The drawing under review shows one solid part. Ordinate dimensions are in mm from its lowest x, y, z. Give positions to 0.01 mm unless a question says otherwise; leave off trailing zeros. Loops run counter-clockwise (first coordinate to the right, second up) from the corner with the lowest first, then second, coordinate; pieces in that order, holes last. Notation, with made-up numbers: (-34, -23.75) - (25, -23.75) arc R15 cw to (25, -12.75) - close; hole circle Ø3 at (44, 77). An arc over 180 degrees is marked (long way). Write each question's results on one line, items separated by ' | '.
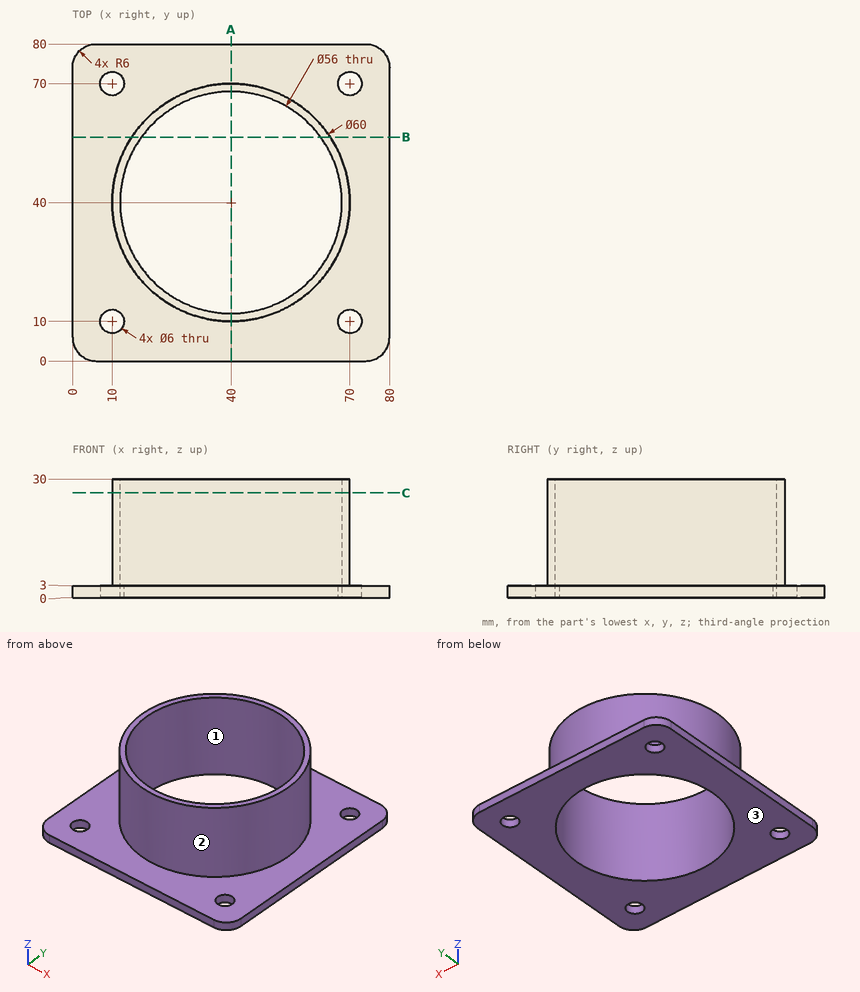
(1) Take a section at A-A on x = 40. Give the boundary of the cut face in (y, z), plus the area to 3 significant figures.
Answers below:
outline: (0, 0) - (12, 0) - (12, 30) - (10, 30) - (10, 3) - (0, 3) - close; (68, 0) - (80, 0) - (80, 3) - (70, 3) - (70, 30) - (68, 30) - close | area: 180 mm2
(2) Insertion check: P1, Ø5, axis at x = 70, y = 34, coming from the -Z side; P2, Ø5, axis at x = 70, y = 10, coming from the -Z side; P3, Ø9.5, axis at x = 10, y = 70, coming from the +Z side; P4, Ø1.5, axis at x = 36.5, z = 23, coming from the -Y side. Each pin has a flat end and moves straight along its axis. Give the tip position at first contact, or say it passes through.
Answers below:
P1: z = 0 | P2: through | P3: z = 3 | P4: y = 10.13
(3) Take a section at C-C on z = 26.5. Give the boundary of the cut face in (x, y).
Answers below:
outline: circle Ø60 at (40, 40); hole circle Ø56 at (40, 40)
(4) Take a section at B-B on y = 56.5. Give the boundary of the cut face in (x, z).
Answers below:
outline: (0, 0) - (17.38, 0) - (17.38, 30) - (14.95, 30) - (14.95, 3) - (0, 3) - close; (62.62, 0) - (80, 0) - (80, 3) - (65.05, 3) - (65.05, 30) - (62.62, 30) - close
(5) Wall thickness on line 1 along Y through (x, z) = (70, 1.3); line 2 along Y through (x, z) = (60, 7.25); line 3 along X through (y, z) = (25, 17.25): over which ranges is each line inside the solid? List them lowest first. Write a range as from..to.
Answers below:
line 1: 0..7, 13..67, 73..80 | line 2: 17.64..20.4, 59.6..62.36 | line 3: 14.02..16.36, 63.64..65.98
(6) Draft analysis for pull direction Y (two halves, no side actions). For the marked faces 1, 2 and 3, state which applies: pulls with the +Y half, pulls with the -Y half, needs draft (parallel to the pull), parting line crosses it, or undercut.
Answers below:
face 1: undercut | face 2: parting line crosses it | face 3: needs draft
